Here's how the part is built. I have some questions about the finished solid (model axes, mm). A direction names the side the tool comes from. Coordinates: 2 decimals unless noted, no trailing zeros. Answer as CSV lines item,"result". Start each with the question number.
```python
from build123d import *

# Parameters (mm, degrees)
BOSS_EXTRUDE3_DEPTH = 206.587093
SHELL1_T            = -3
BOSS_EXTRUDE4_DEPTH = 2
BOSS_EXTRUDE5_DEPTH = 2
SKETCH8_R           = 2.7
CUT_EXTRUDE2_DEPTH  = 3
SKETCH9_R           = 2.7
CUT_EXTRUDE3_DEPTH  = 2
SKETCH11_R          = 2.7
CUT_EXTRUDE4_DEPTH  = 2


with BuildPart() as part:
    # Sketch1 → Boss-Extrude3 (new body)
    with BuildSketch(Plane.XY):
        with BuildLine():
            Line((244.319092767, 234.634840909), (41.119092767, 234.634840909))
            Line((41.119092767, 234.634840909), (41.119092767, 201.934840909))
            Line((41.119092767, 201.934840909), (0, 201.934840909))
            Line((0, 201.934840909), (0, 101.672858907))
            Line((0, 101.672858907), (-12.7, 101.672858907))
            Line((-12.7, 101.672858907), (-12.7, -101.527141093))
            add(Edge.make_bspline(
                [(-12.7, -101.527141093), (212.797902698, -15.185130796), (244.319092767, 234.634840909)],
                knots=[0, 0, 0, 1, 1, 1], degree=2))
        make_face()
    extrude(amount=BOSS_EXTRUDE3_DEPTH)

    # Shell1
    shell1_openings = [part.faces().sort_by_distance(p)[0] for p in [
        (142.719092767, 234.634840909, 103.2935465),
        (-12.7, 0.072858907, 103.2935465),
    ]]
    offset(amount=SHELL1_T, openings=shell1_openings, kind=Kind.INTERSECTION)

    # Sketch4 → Boss-Extrude4 (add)
    with BuildSketch(Plane(origin=(0, 234.634840909, 0), x_dir=(1, 0, 0), z_dir=(0, 1, 0))):
        with BuildLine():
            Line((257.019092767, -10), (257.019092767, -196.587092864))
            ThreePointArc((257.019092767, -196.587092864), (254.090160579, -203.658160676), (247.019092767, -206.587092864))
            Line((247.019092767, -206.587092864), (244.319092767, -206.587092864))
            Line((244.319092767, -206.587092864), (241.295184716, -206.587092864))
            Line((241.295184716, -206.587092864), (241.295184716, 0))
            Line((241.295184716, 0), (247.019092767, 0))
            ThreePointArc((247.019092767, 0), (254.090160579, -2.928932188), (257.019092767, -10))
        make_face()
    extrude(amount=BOSS_EXTRUDE4_DEPTH)

    # Sketch5 → Boss-Extrude5 (add)
    with BuildSketch(Plane.ZY.offset(12.7)):
        with BuildLine():
            Line((10, 114.372858907), (196.587092864, 114.372858907))
            ThreePointArc((196.587092864, 114.372858907), (203.658160676, 111.443926719), (206.587092864, 104.372858907))
            Line((206.587092864, 104.372858907), (206.587092864, 98.672858907))
            Line((206.587092864, 98.672858907), (0, 98.672858907))
            Line((0, 98.672858907), (0, 104.372858907))
            ThreePointArc((0, 104.372858907), (2.928932188, 111.443926719), (10, 114.372858907))
        make_face()
        with BuildLine():
            Line((0, -98.313391167), (0, -101.013391167))
            ThreePointArc((0, -101.013391167), (2.928932188, -108.084458979), (10, -111.013391167))
            Line((10, -111.013391167), (196.587092864, -111.013391167))
            ThreePointArc((196.587092864, -111.013391167), (203.658160676, -108.084458979), (206.587092864, -101.013391167))
            Line((206.587092864, -101.013391167), (206.587092864, -98.313391167))
            Line((206.587092864, -98.313391167), (0, -98.313391167))
        make_face()
    extrude(amount=BOSS_EXTRUDE5_DEPTH)

    # Sketch8 → Cut-Extrude2 (cut)
    with BuildSketch(Plane(origin=(44.119092767, 0, 0), x_dir=(0, 0, -1), z_dir=(1, 0, 0))):
        with Locations(Location((-190.887092864, 211.934840909, 0), (0, 0, 90))):
            Circle(SKETCH8_R)
        with Locations(Location((-103.293546432, 211.934840909, 0), (0, 0, 90))):
            Circle(SKETCH8_R)
        with Locations(Location((-15.7, 211.934840909, 0), (0, 0, 90))):
            Circle(SKETCH8_R)
    extrude(amount=-CUT_EXTRUDE2_DEPTH, mode=Mode.SUBTRACT)

    # Sketch9 → Cut-Extrude3 (cut)
    with BuildSketch(Plane(origin=(0, 236.634840909, 0), x_dir=(1, 0, 0), z_dir=(0, 1, 0))):
        with Locations(Location((249.157138742, -12.931235523, 0), (0, 0, 180))):
            Circle(SKETCH9_R)
        with Locations(Location((249.157138742, -103.293546432, 0), (0, 0, 180))):
            Circle(SKETCH9_R)
        with Locations(Location((249.157138742, -193.655857341, 0), (0, 0, 180))):
            Circle(SKETCH9_R)
    extrude(amount=-CUT_EXTRUDE3_DEPTH, mode=Mode.SUBTRACT)

    # Sketch11 → Cut-Extrude4 (cut)
    with BuildSketch(Plane.ZY.offset(14.7)):
        with Locations(Location((12.933859514, 106.522858907, 0), (0, 0, 270))):
            Circle(SKETCH11_R)
        with Locations(Location((103.293546432, 106.522858907, 0), (0, 0, 270))):
            Circle(SKETCH11_R)
        with Locations(Location((193.653233351, 106.522858907, 0), (0, 0, 270))):
            Circle(SKETCH11_R)
        with Locations(Location((193.728321895, -106.386237609, 0), (0, 0, 270))):
            Circle(SKETCH11_R)
        with Locations(Location((103.368657455, -106.44997351, 0), (0, 0, 270))):
            Circle(SKETCH11_R)
        with Locations(Location((13.008993014, -106.51370941, 0), (0, 0, 270))):
            Circle(SKETCH11_R)
    extrude(amount=-CUT_EXTRUDE4_DEPTH, mode=Mode.SUBTRACT)


solid = part.part
```
1) I need wall thicknesses on line 1 (Z direction, x = 54, y = 135); line 2 (Y direction, x = 37, z = 86); line 3 (X direction, y = 163.5, z = 64). Which ranges of each line are inside material? Lowest first, please. Write a range as [from, to].
2) Will these pins go through, and if not, where does the flat tip stop? pin 1 Ø18 at (y, z) = (210.5, 115) entering from +X; pin 2 Ø7 at (y, z) = (211.93, 190.89) entering from +X; pin 3 Ø2 at (x, z) = (-13.5, 144) entering from +Y; pin 4 Ø1.5 at (x, y) = (44, 152) entering from -Z.
3) Which directions (+Z, -Z, +X, -X, +Y, -Y) give clear straight access to the entire face, cutting with the end or side of a thin tool? Please do faces 1 (the face through (-13.7, 111.5, 203.6)), 2 (the face through (21, 201.935, 102)), 3 (the face through (252, 234.635, 102)).
4) If we mould it in two halves opening along Y, with no side actions, what happens to faces 4 (the face through (-6, 101.673, 102)), 5 (the face through (84, 107, 203.587)), 6 (the face through (-14.7, -103, 102))? For each: released by +Y, released by -Y, zero draft, split by the parting line, or undercut.
Output:
1,line 1,"[0, 3], [203.59, 206.59]"
1,line 2,"[-79.3, -75.92], [198.93, 201.93]"
1,line 3,"[0, 3], [227.43, 230.53]"
2,pin 1,"x = 242.21"
2,pin 2,"x = 241.57"
2,pin 3,"y = 114.37"
2,pin 4,"z = 0"
3,face 1,"+Z, -X, +Y"
3,face 2,"+Z, -Z, -X, +Y"
3,face 3,"+Z, -Z, +X, -Y"
4,face 4,"released by +Y"
4,face 5,"undercut"
4,face 6,"zero draft"
